Input: part model. Units: mm. Frame: model coordinates. A direction names the side the tool comes from. Give positions to 0.01 mm unless a question says otherwise; leave off trailing zeros. Loops run counter-clockwise (first coordinate to the right, second up) from the corner with the lowest first, then second, coordinate; pieces in that order, holes last. Notation, with made-up numbers: (-19.75, 17) -> (0.25, 17) arc R27 cw to (0.25, 42) -> close; hole circle Ø6 at (34, -10). An arc over 180 degrees is marked (long way). Use CSV: the item, a comma, the result in double quotes.
```python
from build123d import *

# Parameters (mm, degrees)
SKETCH1_R           = 45.847
BOSS_EXTRUDE1_DEPTH = 12.7
SKETCH2_R           = 23.876
BOSS_EXTRUDE2_DEPTH = 42.672
SKETCH3_R           = 11.1125
BOSS_EXTRUDE3_DEPTH = 27.305
SKETCH5_R           = 4.7625
CUT_EXTRUDE1_DEPTH  = 25.4
CHAMFER1_SIZE       = 2.54
CHAMFER2_SIZE       = 1.27
SKETCH6_R           = 19.05
CUT_EXTRUDE2_DEPTH  = 50.8
CUT_EXTRUDE3_START  = -2.0574
SKETCH7_R           = 45.847
SKETCH7_R_2         = 43.307
CUT_EXTRUDE3_DEPTH  = 5.08


with BuildPart() as part:
    # Sketch1 → Boss-Extrude1 (new body)
    with BuildSketch(Plane(origin=(0, 0, 0), x_dir=(1, 0, 0), z_dir=(0, 1, 0))):
        with Locations(Location((0, 0, 0), (0, 0, 270))):
            Circle(SKETCH1_R)
    extrude(amount=BOSS_EXTRUDE1_DEPTH)

    # Sketch2 → Boss-Extrude2 (add)
    with BuildSketch(Plane(origin=(0, 12.7, 0), x_dir=(1, 0, 0), z_dir=(0, 1, 0))):
        with Locations(Location((0, 0, 0), (0, 0, 270))):
            Circle(SKETCH2_R)
    extrude(amount=BOSS_EXTRUDE2_DEPTH)

    # Sketch3 → Boss-Extrude3 (add)
    with BuildSketch(Plane(origin=(0, 55.372, 0), x_dir=(1, 0, 0), z_dir=(0, 1, 0))):
        with Locations(Location((0, 0, 0), (0, 0, 270))):
            Circle(SKETCH3_R)
    extrude(amount=BOSS_EXTRUDE3_DEPTH)

    # Sketch5 → Cut-Extrude1 (cut)
    with BuildSketch(Plane(origin=(0, 82.677, 0), x_dir=(1, 0, 0), z_dir=(0, 1, 0))):
        with Locations(Location((0, 0, 0), (0, 0, 270))):
            Circle(SKETCH5_R)
    extrude(amount=-CUT_EXTRUDE1_DEPTH, mode=Mode.SUBTRACT)

    # Chamfer1
    chamfer1_edges = [part.edges().sort_by_distance(p)[0] for p in [
        (0, 82.677, -4.7625),
    ]]
    chamfer(chamfer1_edges, length=CHAMFER1_SIZE)

    # Chamfer2
    chamfer2_edges = [part.edges().sort_by_distance(p)[0] for p in [
        (0, 55.372, -23.876),
    ]]
    chamfer(chamfer2_edges, length=CHAMFER2_SIZE)

    # Sketch6 → Cut-Extrude2 (cut)
    with BuildSketch(Plane.XZ):
        with Locations(Location((0, 0, 0), (0, 0, 270))):
            Circle(SKETCH6_R)
    extrude(amount=-CUT_EXTRUDE2_DEPTH, mode=Mode.SUBTRACT)

    # Sketch7 → Cut-Extrude3 (cut)
    with BuildSketch(Plane.XZ.offset(CUT_EXTRUDE3_START)):
        with Locations(Location((0, 0, 0), (0, 0, 270))):
            Circle(SKETCH7_R)
        with Locations(Location((0, 0, 0), (0, 0, 270))):
            Circle(SKETCH7_R_2, mode=Mode.SUBTRACT)
    extrude(amount=-CUT_EXTRUDE3_DEPTH, mode=Mode.SUBTRACT)


solid = part.part
```
1) Ray query, line 1 (X direction, y = 75.5, z = 0); line 2 (Y direction, x = -37, z = 26); line 3 (Y direction, x = -38, z = 10). Return the intervals inside material, ascending.
From the geometry:
line 1,"x = -11.11 to -4.76, 4.76 to 11.11"
line 2,"y = 0 to 2.06, 7.14 to 12.7"
line 3,"y = 0 to 12.7"
2) Section query C-C (y = 62.5). Return loops of the section in (x, z) (1 decimal), then the cut area to 3 significant figures.
From the geometry:
outline,"circle Ø22.2 at (0, 0); hole circle Ø9.5 at (0, 0)"
area,"317 mm^2"
3) Reachability of faces 4 (the cylindrical face through (42.94, 4.56, 5.64)), 5 (the cylindrical face through (13.77, 9.88, 43.73)), 6 (the flat face through (0, 50.8, 0)), 7 (the flat face through (1, 0, 20)), 8 (the flat face through (10.4, 55.372, 4.7)) from +Z, -Z, +X, -X, +Y, -Y: full face, straight path, thin tool, end or side. Return the list, or none.
From the geometry:
face 4,"none"
face 5,"+Y, -Y"
face 6,"-Y"
face 7,"+Z, -Z, +X, -X, -Y"
face 8,"+Y"
4) Mould query, pull axis X, two halves, no side actions, for faces 1 (the cylindrical face through (7.172, 33.111, 22.773)), 2 (the flat face through (0, 57.277, 0)), 3 (the flat face through (-33.75, 7.137, 27.38)). Classes: pulls with the +X half, pulls with the -X half, needs draft (parallel to the pull), parting line crosses it, or undercut.
From the geometry:
face 1,"parting line crosses it"
face 2,"undercut"
face 3,"needs draft"
5) Section query D-D (z = -30.5). Return loops of the section in (x, y), then the cut area to 3 significant figures.
From the geometry:
outline,"(-34.23, 0) -> (34.23, 0) -> (34.23, 2.06) -> (30.74, 2.06) -> (30.74, 7.14) -> (34.23, 7.14) -> (34.23, 12.7) -> (-34.23, 12.7) -> (-34.23, 7.14) -> (-30.74, 7.14) -> (-30.74, 2.06) -> (-34.23, 2.06) -> close"
area,"834 mm^2"
6) Contact query for flat-ended pins moving along their axis: pin 1 (1.5 mm diameter, centred on x = 15, z = -33, fed in from +Y); pin 2 (12 mm diameter, centred on y = 48, z = -14, fed in from -X); pin 3 (6 mm diameter, centred on y = 55, z = -24.5, fed in from -X); pin 4 (13.5 mm diameter, centred on x = -0.5, z = -5.5, fed in from +Y). Output: stop coordinate, or through.
From the geometry:
pin 1,"stops at y = 12.7"
pin 2,"stops at x = -22.5"
pin 3,"stops at x = -10.09"
pin 4,"stops at y = 82.68"
